Autodesk Inventor part; units mm, degrees
ref_plane "YZ Plane" through (0, 0, 0) normal (1, 0, 0) x (0, 1, 0)
ref_plane "XZ Plane" through (0, 0, 0) normal (0, 1, 0) x (-1, 0, 0)
ref_plane "XY Plane" through (0, 0, 0) normal (0, 0, 1) x (1, 0, 0)
sketch "Sketch1" plane through (0, 0, 0) normal (0, 1, 0) x (-1, 0, 0)
  circle A0 centre (0, 0) radius 51.435
  circle A1 centre (0, 0) radius 60.198
  dimension "d0" = 102.87
  dimension "d1" = 120.396
extrude "Extrusion1" add sketch "Sketch1" along normal blind 5.08
sketch "Sketch2" plane through (0, 5.08, 0) normal (0, 1, 0) x (1, 0, 0)
  circle A0 centre (0, 0) radius 55.245
  point P0 (-55.245, 0)
  point P1 (-27.6225, -47.8436)
  point P2 (27.6225, -47.8436)
  point P3 (55.245, 0)
  point P4 (27.6225, 47.8436)
  point P5 (-27.6225, 47.8436)
  dimension "d4" = 110.49
  dimension "d8" = 360
hole "Hole1" at (-55.245, 5.08, 0) at (-27.6225, 5.08, 47.8436) at (27.6225, 5.08, 47.8436) at (55.245, 5.08, 0) at (27.6225, 5.08, -47.8436) at (-27.6225, 5.08, -47.8436) direction (0, -1, 0) diameter 3 end through all
chamfer "Chamfer1" distance 0.508 angle 45 1 edges at (60.198, 0, 0)
properties part number "Oring Fitting Dome V2 -part"
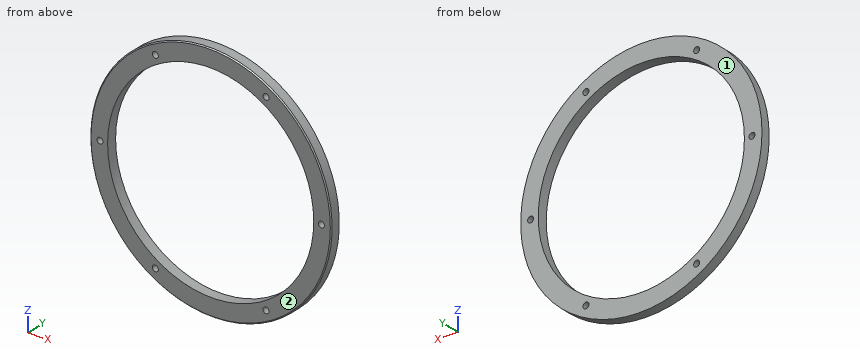
Build history of the part. All positions in model axes, mm. Face numbers are marked on the shaded views. Round coordinates to 2 decimals unless told otherwise and drop trailing zeros. Loops run counter-clockwise (first coordinate to the right, second up) from the corner with the lowest first, then second, coordinate; pieces in that order, holes last. Notation, with made-up numbers: M 3,25 L 7,25 A25 ccw 7,55 Z; hole C 15,49.5 d9. An arc over 180 degrees is marked long. Answer as CSV lines item,"result".
1. Cut at A-A on x = 0. Write the cut outline in (y, z) (3 decimals), then the cut area to 3 significant figures.
Resolved:
outline,"M 0,-59.69 L 0.508,-60.198 L 5.08,-60.198 L 5.08,-51.435 L 0,-51.435 Z; M 0,51.435 L 5.08,51.435 L 5.08,60.198 L 0.508,60.198 L 0,59.69 Z"
area,"88.8 mm²"
2. Two-plate mould, pull along Y, no slides. Class the marked faces 1 and 2: released by +Y, released by -Y, zero draft, split by the parting line, or undercut.
Resolved:
face 1,"released by +Y"
face 2,"released by -Y"
3. Cut at B-B on z = 0. Write the cut outline in (x, y) (3 decimals).
Resolved:
outline,"M -60.198,0.508 L -59.69,0 L -56.745,0 L -56.745,5.08 L -60.198,5.08 Z; M -53.745,0 L -51.435,0 L -51.435,5.08 L -53.745,5.08 Z; M 51.435,0 L 53.745,0 L 53.745,5.08 L 51.435,5.08 Z; M 56.745,0 L 59.69,0 L 60.198,0.508 L 60.198,5.08 L 56.745,5.08 Z"
4. Cut at C-C on y = 3.35. Write the cut outline in (x, z) (1 decimal).
Resolved:
outline,"C 0,0 d120.4; hole C -55.2,0 d3; hole C 0,0 d102.9; hole C -27.6,-47.8 d3; hole C -27.6,47.8 d3; hole C 27.6,-47.8 d3; hole C 27.6,47.8 d3; hole C 55.2,0 d3"
5. Flat gauge pins, fed straight in: P1, Ø2, axis at x = 9.5, y = 2, coming from the -Z side; P2, Ø1, axis at x = 41.5, y = 3.5, coming from the -Z side; P3, Ø1.8, axis at x = -27.62, z = -47.84, coming from the +Y side; P4, Ø1, axis at x = -1, y = 3.5, coming from the -Z side. Where does each tip first touch, or does it go through?
Resolved:
P1,"stops at z = -59.59"
P2,"stops at z = -44.08"
P3,"passes through"
P4,"stops at z = -60.2"
6. Wall check: probe 1 along X at (y, z) = (3.3, 47.5); probe 2 along X at (y, z) = (3.15, 0.5); probe 3 along Z at (x, y) = (-26.5, 4). Give the ranges that are in metal, low to high. Write a range as [from, to].
Resolved:
probe 1,"x = [-36.98, -29.08], [-26.16, -19.73], [19.73, 26.16], [29.08, 36.98]"
probe 2,"x = [-60.2, -56.66], [-53.83, -51.43], [51.43, 53.83], [56.66, 60.2]"
probe 3,"z = [-54.05, -48.84], [-46.85, -44.08], [44.08, 46.85], [48.84, 54.05]"
